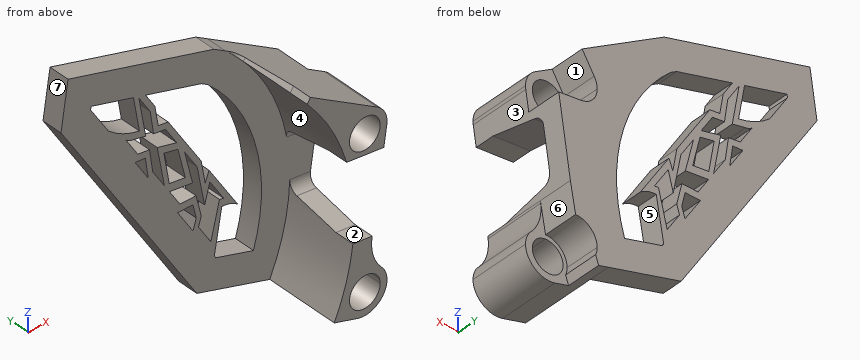
from build123d import *

# Parameters (mm, degrees)
F1_DEPTH = 6.096
F0_R     = 4.7625
F2_DEPTH = 27.94
F3_R     = 4.7625
F4_DEPTH = 10.16
F6_DEPTH = 25.4
F8_DEPTH = 25.4


# Not quite as in the source:
# - ends of sketch curves that miss each other by under 0.0002 mm in the source are joined


with BuildPart() as f1:
    # F0 (on Front) → F1 (new body)
    with BuildSketch(Plane.XZ):
        with BuildLine():
            Line((-32.0214776694, -42.0687062724), (-9.4581565389, -49.9383443038))
            ThreePointArc((-9.4581565389, -49.9383443038), (-4.3291887886, -10.8925785557), (-23.2082019061, 23.6683964993))
            Line((-23.2082019061, 23.6683964993), (-26.7419346225, 26.0181961702))
            Line((-26.7419346225, 26.0181961702), (-71.8849952467, 41.1920125155))
            Line((-71.8849952467, 41.1920125155), (-74.0636416555, 26.7504224083))
            Line((-74.0636416555, 26.7504224083), (-32.0214776694, -42.0687062724))
        make_face()
        with BuildLine():
            Line((-64.9229101249, 28.5970199237), (-64.7778869932, 29.5583345343))
            Line((-64.7778869932, 29.5583345343), (-51.6396961272, 25.1422295438))
            Line((-51.6396961272, 25.1422295438), (-52.8126453404, 31.9232999149))
            Line((-52.8126453404, 31.9232999149), (-47.9094184009, 23.888381259))
            Line((-47.9094184009, 23.888381259), (-30.6306738726, 18.0805230295))
            Line((-30.6306738726, 18.0805230295), (-28.7005674828, 16.7970746978))
            ThreePointArc((-28.7005674828, 16.7970746978), (-13.7073707997, -9.0370384003), (-14.5091616555, -38.895947921))
            Line((-14.5091616555, -38.895947921), (-26.1770067548, -34.8264354141))
            Line((-26.1770067548, -34.8264354141), (-26.621853962, -34.0982617358))
            Line((-26.621853962, -34.0982617358), (-26.6298627107, -34.143893025))
            Line((-26.6298627107, -34.143893025), (-33.2056261218, -23.3681886247))
            Line((-33.2056261218, -23.3681886247), (-33.1959865258, -23.3370155967))
            Line((-33.1959865258, -23.3370155967), (-37.9909119068, -15.4881668334))
            Line((-37.9909119068, -15.4881668334), (-38.0149602805, -15.4871320814))
            Line((-38.0149602805, -15.4871320814), (-47.058612277, -0.6672983188))
            Line((-47.058612277, -0.6672983188), (-47.0628196228, -0.6382941035))
            Line((-47.0628196228, -0.6382941035), (-51.126360936, 6.0133466785))
            Line((-51.126360936, 6.0133466785), (-51.1360904547, 6.0144657282))
            Line((-51.1360904547, 6.0144657282), (-59.3956089847, 19.549339872))
            Line((-59.3956089847, 19.549339872), (-64.9229101249, 28.5970199237))
        make_face(mode=Mode.SUBTRACT)
        Polygon((-52.8126453404, 31.9232999149), (-51.6396961272, 25.1422295438), (-47.9094184009, 23.888381259), align=None)
        with BuildLine():
            Line((-47.9094184009, 23.888381259), (-51.6396961272, 25.1422295438))
            Line((-51.6396961272, 25.1422295438), (-49.7922885775, 14.4619712189))
            ThreePointArc((-49.7922885775, 14.4619712189), (-54.9303785287, 16.3705840809), (-59.3956089847, 19.549339872))
            Line((-59.3956089847, 19.549339872), (-51.126360936, 6.0133466785))
            Line((-51.126360936, 6.0133466785), (-47.9751295821, 5.650904873))
            Line((-47.9751295821, 5.650904873), (-47.0628196228, -0.6382941035))
            Line((-47.0628196228, -0.6382941035), (-37.9909119068, -15.4881668334))
            Line((-37.9909119068, -15.4881668334), (-33.2459525636, -15.6923326562))
            Line((-33.2459525636, -15.6923326562), (-32.1973996311, -20.1077332485))
            Line((-32.1973996311, -20.1077332485), (-33.1959865258, -23.3370155967))
            Line((-33.1959865258, -23.3370155967), (-26.621853962, -34.0982617358))
            Line((-26.621853962, -34.0982617358), (-24.3119723824, -20.937295163))
            ThreePointArc((-24.3119723824, -20.937295163), (-21.7000142249, -21.4617233548), (-19.4071664649, -22.8182628838))
            Line((-19.4071664649, -22.8182628838), (-28.2510661679, -8.3257632317))
            Line((-28.2510661679, -8.3257632317), (-29.4364036114, -11.4075290833))
            Line((-29.4364036114, -11.4075290833), (-30.6980011467, -4.3159705476))
            Line((-30.6980011467, -4.3159705476), (-40.9051855797, 12.4105439777))
            Line((-40.9051855797, 12.4105439777), (-43.9856683867, 12.9511995939))
            Line((-43.9856683867, 12.9511995939), (-45.0197701825, 19.1531143287))
            Line((-45.0197701825, 19.1531143287), (-47.9094184009, 23.888381259))
        make_face()
        Polygon((-27.6263519566, -29.1291445767), (-27.7209985719, -29.3173462139), (-31.515369772, -23.0995096098), (-30.6589124026, -20.3298531285), (-32.2562875166, -13.6033915394), (-37.2546680921, -13.3883215232), (-40.5128122557, -8.0492002372), (-33.339172628, -9.3082459116), (-35.8258069544, 1.0090607264), (-31.9595713249, -5.326540128), (-29.5939579287, -17.6900622221), (-28.0038996356, -11.8086998658), (-23.7145710116, -18.8376232681), (-25.0080493325, -18.5184438136), align=None, mode=Mode.SUBTRACT)
        Polygon((-42.2277428728, 4.0048563327), (-37.873417838, 2.8701371118), (-35.5923646419, -6.559544504), (-40.5642118698, -5.6869354699), align=None, mode=Mode.SUBTRACT)
        with BuildLine():
            Line((-46.4479878328, 18.3739303005), (-45.4261892475, 11.3299486454))
            Line((-45.4261892475, 11.3299486454), (-41.7172805078, 10.6789979777))
            Line((-41.7172805078, 10.6789979777), (-38.2356426654, 4.9736375696))
            Line((-38.2356426654, 4.9736375696), (-44.2720463387, 6.7649825752))
            Line((-44.2720463387, 6.7649825752), (-42.0774568025, -5.4481170908))
            Line((-42.0774568025, -5.4481170908), (-45.6646201437, 0.4301679667))
            Line((-45.6646201437, 0.4301679667), (-46.6726678742, 7.3793552358))
            Line((-46.6726678742, 7.3793552358), (-50.293044526, 8.0147676345))
            Line((-50.293044526, 8.0147676345), (-53.9911477917, 14.0748499614))
            ThreePointArc((-53.9911477917, 14.0748499614), (-53.0287307311, 13.4025301345), (-51.9140375876, 13.0341285278))
            Line((-51.9140375876, 13.0341285278), (-47.8512962747, 11.9523388206))
            Line((-47.8512962747, 11.9523388206), (-49.9565863421, 24.1234711571))
            Line((-49.9565863421, 24.1234711571), (-46.4479878328, 18.3739303005))
        make_face(mode=Mode.SUBTRACT)
        Polygon((-37.9909119068, -15.4881668334), (-47.0628196228, -0.6382941035), (-47.058612277, -0.6672983188), (-38.0149602805, -15.4871320814), align=None)
        Polygon((-26.621853962, -34.0982617358), (-33.1959865258, -23.3370155967), (-33.2056261218, -23.3681886247), (-26.6298627107, -34.143893025), align=None)
        Polygon((-51.126360936, 6.0133466785), (-59.3956089847, 19.549339872), (-51.1360904547, 6.0144657282), align=None)
    extrude(amount=F1_DEPTH)

    # F0 (on Front) → F2 (join)
    with BuildSketch(Plane.XZ):
        with BuildLine():
            ThreePointArc((-2.2585047177, -52.4494397874), (-6.6570778662, -44.3261291668), (1.0230165746, -39.1927316018))
            Line((1.0230165746, -39.1927316018), (2.1631019861, -31.6354491837))
            ThreePointArc((2.1631019861, -31.6354491837), (2.210106245, -31.292191847), (2.2664563284, -30.9503444137))
            Line((2.2664563284, -30.9503444137), (6.781268444, -1.0230162708))
            ThreePointArc((6.781268444, -1.0230162708), (-6.2699855461, -2.7783889669), (3.7973937006, 5.7106886698))
            Line((3.7973937006, 5.7106886698), (-23.2082019061, 23.6683964993))
            ThreePointArc((-23.2082019061, 23.6683964993), (-4.3291887886, -10.8925785557), (-9.4581565389, -49.9383443038))
            Line((-9.4581565389, -49.9383443038), (-2.2585047177, -52.4494397874))
        make_face()
        with BuildLine():
            ThreePointArc((3.7973937006, 5.7106886698), (-6.2699855461, -2.7783889669), (6.781268444, -1.0230162708))
            ThreePointArc((6.781268444, -1.0230162708), (6.8387902069, -0.5129449342), (6.858, 0))
            ThreePointArc((6.858, 0), (6.0446128908, 3.239570805), (3.7973937006, 5.7106886698))
        make_face()
        Circle(F0_R, mode=Mode.SUBTRACT)
        with BuildLine():
            Line((2.1631019861, -31.6354491837), (1.0230165746, -39.1927316018))
            ThreePointArc((1.0230165746, -39.1927316018), (3.1078508959, -39.8606190362), (4.8759932113, -41.1514639241))
            ThreePointArc((4.8759932113, -41.1514639241), (2.5546345778, -36.6685406241), (2.1631019861, -31.6354491837))
        make_face()
        with BuildLine():
            ThreePointArc((4.8759932113, -41.1514639241), (3.1078508959, -39.8606190362), (1.0230165746, -39.1927316018))
            ThreePointArc((1.0230165746, -39.1927316018), (-6.6570778662, -44.3261291668), (-2.2585047177, -52.4494397874))
            ThreePointArc((-2.2585047177, -52.4494397874), (3.9713561063, -51.5651085374), (6.858, -45.974))
            ThreePointArc((6.858, -45.974), (6.3431744987, -43.3670283318), (4.8759932113, -41.1514639241))
        make_face()
        with BuildLine():
            ThreePointArc((0.7104281768, -41.2647858346), (3.6100429666, -42.8677166857), (4.7625, -45.974))
            ThreePointArc((4.7625, -45.974), (-3.6100429666, -49.0802833143), (0.7104281768, -41.2647858346))
        make_face(mode=Mode.SUBTRACT)
    extrude(amount=F2_DEPTH)

    # F3 (on face) → F4 (cut)
    with BuildSketch(Plane(origin=(0, 0, 0), x_dir=(-1, 0, 0), z_dir=(0, 1, 0))):
        with BuildLine():
            ThreePointArc((1.0479234506, -5.9407838449), (4.6212906458, -3.8774642509), (6.0325, 0))
            ThreePointArc((6.0325, 0), (5.7966808552, 1.6701937951), (5.1076604432, 3.2098070109))
            ThreePointArc((5.1076604432, 3.2098070109), (-5.5141755069, 2.4464105806), (1.0479234506, -5.9407838449))
        make_face()
        Circle(F3_R, mode=Mode.SUBTRACT)
        with BuildLine():
            ThreePointArc((1.0479234506, -5.9407838449), (-5.5141755069, 2.4464105806), (5.1076604432, 3.2098070109))
            Line((5.1076604432, 3.2098070109), (1.3747032796, 9.1499391047))
            Line((1.3747032796, 9.1499391047), (-3.7973937006, 5.7106886698))
            ThreePointArc((-3.7973937006, 5.7106886698), (-6.2699855461, 2.7783889669), (-6.781268444, -1.0230162708))
            Line((-6.781268444, -1.0230162708), (-5.8556681398, -7.158541587))
            Line((-5.8556681398, -7.158541587), (1.0479234506, -5.9407838449))
        make_face()
        with BuildLine():
            Line((-0.6517694903, -39.9768129276), (-2.2664563284, -30.9503444137))
            ThreePointArc((-2.2664563284, -30.9503444137), (-2.46420133, -36.3340905871), (-4.8759932113, -41.1514639241))
            ThreePointArc((-4.8759932113, -41.1514639241), (-5.7986098468, -49.6357329019), (2.2585047177, -52.4494397874))
            Line((2.2585047177, -52.4494397874), (6.4636236378, -50.9827778723))
            Line((6.4636236378, -50.9827778723), (5.5451457053, -48.3493768874))
            ThreePointArc((5.5451457053, -48.3493768874), (-4.8488389859, -49.5628461571), (-0.6517694903, -39.9768129276))
        make_face()
        with BuildLine():
            ThreePointArc((6.0325, -45.974), (4.0286012957, -41.483852135), (-0.6517694903, -39.9768129276))
            ThreePointArc((-0.6517694903, -39.9768129276), (-4.8488389859, -49.5628461571), (5.5451457053, -48.3493768874))
            ThreePointArc((5.5451457053, -48.3493768874), (5.9094055419, -47.1864283036), (6.0325, -45.974))
        make_face()
        with Locations((0, -45.974)):
            Circle(F3_R, mode=Mode.SUBTRACT)
        with Locations((0, -45.974)):
            Circle(F3_R)
    extrude(amount=-F4_DEPTH, mode=Mode.SUBTRACT)

    # F5 (on face) → F6 (cut)
    with BuildSketch(Plane(origin=(6.7812683982, 0, -1.0230165746), x_dir=(0, 1, 0), z_dir=(0.9888113733, 0, -0.1491712707))):
        with BuildLine():
            Line((-27.94, -6.1359623937), (-27.94, -30.2659623937))
            Line((-27.94, -30.2659623937), (-22.225, -30.2659623937))
            Line((-22.225, -30.2659623937), (-8.6577684612, -27.5952475238))
            ThreePointArc((-8.6577684612, -27.5952475238), (-6.81869138, -26.496664003), (-6.096, -24.4800313066))
            Line((-6.096, -24.4800313066), (-6.096, -18.2009623937))
            Line((-6.096, -18.2009623937), (-6.096, -11.9218934807))
            ThreePointArc((-6.096, -11.9218934807), (-6.81869138, -9.9052607843), (-8.6577684612, -8.8066772635))
            Line((-8.6577684612, -8.8066772635), (-22.225, -6.1359623937))
            Line((-22.225, -6.1359623937), (-27.94, -6.1359623937))
        make_face()
    extrude(amount=-F6_DEPTH, mode=Mode.SUBTRACT)

    # F7 (on face) → F8 (cut)
    with BuildSketch(Plane(origin=(3.7973937006, 0, 5.7106886698), x_dir=(0.8327046763, 0, -0.5537173667), z_dir=(0.5537173667, 0, 0.8327046763))):
        with BuildLine():
            Line((-32.4311804374, -6.096), (-32.4311804374, -27.94))
            Line((-32.4311804374, -27.94), (-24.8111804374, -27.94))
            Line((-24.8111804374, -27.94), (-24.8111804374, -22.225))
            Line((-24.8111804374, -22.225), (-27.8331080585, -8.5842698128))
            ThreePointArc((-27.8331080585, -8.5842698128), (-28.9454580871, -6.7950160194), (-30.9329510626, -6.096))
            Line((-30.9329510626, -6.096), (-32.4311804374, -6.096))
        make_face()
    extrude(amount=-F8_DEPTH, mode=Mode.SUBTRACT)


solid = f1.part
Geometry: final body of the model. Coordinates: model frame, mm. Face numbers are marked on the shaded views. A direction names the side the tool comes from. Coordinates: 2 decimals unless noted, no trailing zeros. Order: outer loops, then holes, each group sorted by start corner. A loop starts at its lowest first (then second) coordinate and runs counter-clockwise, first axis right, second up.
(1) First-contact query: pin 1 (10 mm diameter, centred on y = -8.5, z = -41.5, fed in from -X); pin 2 (3 mm diameter, centred on y = -9.5, z = 29, fed in from +X); pin 3 (10 mm diameter, centred on x = -13.5, y = -20.5, fed in from +Z); pin 4 (2 mm diameter, centred on y = -18, z = 9, fed in from -X). Flat tips, straight axial feed; report the tip coordinate or a pass-through.
(2) Section query B-B (x = -66). Return the cut outline in (y, z), plus the area to 3 significant figures.
(3) Material intervals for probe 1 along Z at (x, y) = (0, -14.5); probe 2 along Z at (x, y) = (0, -23.75); probe 3 along X at (y, z) = (-11.75, -42.5), sorted ascending.
(4) Access query for the marked faces 1, 2, 3 and 4. Directions: +Z, -Z, +X, -X, +Y, -Y. A direction counts if a zero-diameter tool reaches every point of the face in a straight line with its end or side. Return the directions, or none.
(5) Section query A-A (y = -18.25). Return the cut outline in (x, z) (1 decimal), plus the area to 3 significant figures.
(6) Draft query along Z for the marked faces 5, 6 and 7. Return one class per face: pulls with the +Z half, pulls with the -Z half, needs draft (parallel to the pull), parting line crosses it, or undercut.
Solution:
1. pin 1: stops at x = -35.05
1. pin 2: passes through
1. pin 3: stops at z = 20
1. pin 4: stops at x = -12.23
2. outline: (-6.1, 13.55) - (0, 13.55) - (0, 39.21) - (-6.1, 39.21) - close
2. area: 156 mm2
3. probe 1: z = -52.83 to -50.74, -41.21 to -29.07, -7.74 to -4.76, 4.76 to 8.24
3. probe 2: z = -52.83 to -50.74, -41.21 to -30.61, -6.21 to -4.76, 4.76 to 8.24
3. probe 3: x = -6.46 to -3.26, 3.26 to 5.91
4. face 1: +X, +Y
4. face 2: +X, -Y
4. face 3: +X, +Y, -Y
4. face 4: -X, -Y
5. outline: (-18.4, 18.7) arc R63.5 cw to (-5.4, -6.2) - (5.7, -7.9) - (6.8, -1) arc R6.9 ccw to (3.8, 5.7) - (-17.6, 19.9) - close; (-9.5, -49.9) - (-2.3, -52.4) arc R6.9 ccw to (4.9, -41.2) arc R12.7 cw to (2.3, -31) - (2.4, -30.2) - (-3.6, -29.3) arc R63.5 cw to start; hole circle Ø9.5 at (0, -46); hole circle Ø9.5 at (0, 0)
5. area: 366 mm2
6. face 5: undercut
6. face 6: pulls with the -Z half
6. face 7: pulls with the +Z half
